from build123d import *

# Parameters (mm, degrees)
F1_DEPTH = 38.1
F3_DEPTH = 12.7
F4_W     = 37.890759
F4_H     = 8.996059
F5_DEPTH = 25.4
F7_DEPTH = 25.4


with BuildPart() as f1:
    # F0 (on Top) → F1 (new body)
    with BuildSketch(Plane.XY):
        with BuildLine():
            Line((-12.425475, 27.331422), (-12.425475, 36.439589))
            ThreePointArc((-12.425475, 36.439589), (-38.49982, 0), (-12.425475, -36.439589))
            Line((-12.425475, -36.439589), (-12.425475, -27.331422))
            ThreePointArc((-12.425475, -27.331422), (-30.023308, 0), (-12.425475, 27.331422))
        make_face()
        with BuildLine():
            ThreePointArc((-12.425475, -36.439589), (22.403767, -31.30986), (38.49982, 0))
            ThreePointArc((38.49982, 0), (22.403767, 31.30986), (-12.425475, 36.439589))
            Line((-12.425475, 36.439589), (-12.425475, 27.331422))
            ThreePointArc((-12.425475, 27.331422), (16.253387, 25.243345), (30.023308, 0))
            ThreePointArc((30.023308, 0), (16.253387, -25.243345), (-12.425475, -27.331422))
            Line((-12.425475, -27.331422), (-12.425475, -36.439589))
        make_face()
    extrude(amount=F1_DEPTH)

    # F2 (on Top) → F3 (join)
    with BuildSketch(Plane.XY):
        with BuildLine():
            ThreePointArc((-8.232961, -37.371887), (-38.267997, 0), (-8.232961, 37.371887))
            Line((-8.232961, 37.371887), (-8.232961, 37.649773))
            Line((-8.232961, 37.649773), (-95.211737, 37.649773))
            Line((-95.211737, 37.649773), (-95.211737, -37.371887))
            Line((-95.211737, -37.371887), (-8.232961, -37.371887))
        make_face()
    extrude(amount=F3_DEPTH)

    # F4 (on face) → F5 (join)
    with BuildSketch(Plane.XY.offset(12.7)):
        with Locations((-57.37193, -2.123943)):
            Rectangle(F4_W, F4_H)
    extrude(amount=F5_DEPTH)

    # F6 (on face) → F7 (cut)
    with BuildSketch(Plane(origin=(0, 2.374087, 0), x_dir=(-1, 0, 0), z_dir=(0, 1, 0))):
        Polygon((76.31731, 38.1), (38.426551, 38.1), (76.31731, 12.7), align=None)
    extrude(amount=-F7_DEPTH, mode=Mode.SUBTRACT)


solid = f1.part
Can you work these out from the model? Positions are in its coordinate system, mm. A direction names the side the tool comes from. Coordinates: 2 decimals unless noted, no trailing zeros. Order: outer loops, then holes, each group sorted by start corner. A loop starts at its lowest first (then second) coordinate and runs counter-clockwise, first axis right, second up. Notation, with made-up numbers: (24, 30.25) - (53, 30.25) arc R15 ccw to (53, 48.25) - close; hole circle Ø4 at (39.5, 57). An arc over 180 degrees is marked (long way). Answer as a JSON object with one key per item and string values. Group by question number.
Q1. Imagine slicing it at B-B (y = 23). Please give me the cut outline in (x, z).
Q2. Imagine slicing it at A-A (x = -2.5). Please give me the cut outline in (y, z), and give its area (3 significant figures).
Q3. On a 3-axis mill with a long thin cutter (end or side, diameter ignored), from which of +Z, -Z, +X, -X, +Y, -Y can I reach the whole of each face in a straight line? I mean faces 1 (the face through (-53, -37.372, 6)), 2 (the face through (-53, 2.374, 20)), 3 (the face through (-53, -6.622, 22)), 4 (the face through (-51, 37.65, 6)). Say none if no direction works.
Q4. I need wall thicknesses on line 1 (Y direction, x = 1, z = 22); line 2 (Y direction, x = -59.5, z = 9); line 3 (Z direction, x = -81.5, y = -15.5). Which ranges of each line are inside material? Lowest first, please. Write a range as from..to.
Q5. Will these pins go through, and if not, where does the flat tip stop? P1, Ø6, axis at y = -21.5, z = 9, coming from the +X side; P2, Ø1, axis at x = -73.5, z = 8.5, coming from the -Y side; P3, Ø4, axis at x = -7, z = 27.5, coming from the +Y side.
Q6. Imagine slicing it at D-D (x = -35). Please give me the cut outline in (y, z).
Q7. Imagine slicing it at C-C (z = 4.5). Please give me the cut outline in (x, y), and give its area (3 significant figures).
Determined:
{
 "1": {"outline": "(-95.21, 0) - (-19.3, 0) - (-19.3, 38.1) - (-30.87, 38.1) - (-30.87, 12.7) - (-95.21, 12.7) - close; (19.3, 0) - (30.87, 0) - (30.87, 38.1) - (19.3, 38.1) - close"},
 "2": {"outline": "(-38.42, 0) - (-29.92, 0) - (-29.92, 38.1) - (-38.42, 38.1) - close; (29.92, 0) - (38.42, 0) - (38.42, 38.1) - (29.92, 38.1) - close", "area": "648 mm2"},
 "3": {"face 1": "+Z, -Z, -X, -Y", "face 2": "+Z, -X, +Y", "face 3": "+Z, -X, -Y", "face 4": "+Z, -Z, -X, +Y"},
 "4": {"line 1": "y = -38.49..-30.01, 30.01..38.49", "line 2": "y = -37.37..37.65", "line 3": "z = 0..12.7"},
 "5": {"P1": "stops at x = 33.76", "P2": "stops at y = -37.37", "P3": "stops at y = 38.17"},
 "6": {"outline": "(-37.37, 0) - (37.65, 0) - (37.65, 12.7) - (16.04, 12.7) - (16.04, 38.1) - (-16.04, 38.1) - (-16.04, 12.7) - (-37.37, 12.7) - close"},
 "7": {"outline": "(-95.21, -37.37) - (-9.25, -37.37) arc R38.5 ccw (long way) to (-8.23, 37.61) - (-8.23, 37.65) - (-95.21, 37.65) - close; hole (-12.43, 27.33) arc R30.02 ccw (long way) to (30.02, 0) arc R30.02 ccw to start", "area": "6,650 mm2"}
}
